Part model, mm, in its own coordinate system. Coordinates: 2 decimals unless noted, no trailing zeros. Order: outer loops, then holes, each group sorted by start corner. A loop starts at its lowest first (then second) coordinate and runs counter-clockwise, first axis right, second up.
```python
from build123d import *

# Parameters (mm, degrees)
SKETCH1_W           = 127
SKETCH1_H           = 63.5
BOSS_EXTRUDE1_DEPTH = 2.286
SKETCH2_R           = 3.3734375
CUT_EXTRUDE1_DEPTH  = 143.008717324
CHAMFER1_SIZE       = 20.32


with BuildPart() as part:
    # Sketch1 → Boss-Extrude1 (new body)
    with BuildSketch(Plane(origin=(0, 0, 0), x_dir=(1, 0, 0), z_dir=(0, 1, 0))):
        with Locations((63.5, 31.75)):
            Rectangle(SKETCH1_W, SKETCH1_H)
    extrude(amount=BOSS_EXTRUDE1_DEPTH)

    # Sketch2 → Cut-Extrude1 (cut, through all)
    with BuildSketch(Plane(origin=(0, 2.286, 0), x_dir=(1, 0, 0), z_dir=(0, 1, 0))):
        with Locations(Location((25.4, 25.4, 0), (0, 0, 270))):
            Circle(SKETCH2_R)
        with Locations(Location((101.6, 25.4, 0), (0, 0, 270))):
            Circle(SKETCH2_R)
    extrude(amount=-CUT_EXTRUDE1_DEPTH, mode=Mode.SUBTRACT)

    # Chamfer1
    chamfer1_edges = [part.edges().sort_by_distance(p)[0] for p in [
        (0, 1.143, -63.5),
        (127, 1.143, -63.5),
    ]]
    chamfer(chamfer1_edges, length=CHAMFER1_SIZE)


solid = part.part
```
(1) Slice it at A-A, the plane x = 101.6. Give the cut face in (y, z).
(2) Drop a flat-ended pin along its axis: pin 1 (9 mm diameter, centred on x = 25.4, z = -25.4, fed in from -Y). Give the stop position or say it passes through.
(3) Slice it at B-B, the plane z = -25.4. Give the cut face in (x, y), then the cut area to 3 significant figures.
(4) Slice it at D-D, the plane z = -47. Give the cut face in (x, y).
(5) Slice it at C-C, the plane y = 0.45. Give the cut face in (x, z), then the cut area to 3 significant figures.
(6) Pull direction Z, two halves, no side cores. Call faces 1 (the face through (63, 1, 0)), 2 (the face through (10.3, 1.13, -53.48)), 3 (the face through (63, 2.286, -32)), 4 (the face through (25.55, 1.16, -28.77)): +Z half, -Z half, draft (parallel to the pull), parting line (faces both ways), or undercut.
(7) Probe line 1 (X direction, y = 0.7, z = -25.4); line 2 (X direction, y = 1.6, z = -23); line 3 (Z direction, x = 100.5, y = 2). List the from-to ranges inside material, lowest first.
Here are the results:
1. outline: (0, -63.5) - (2.29, -63.5) - (2.29, -28.77) - (0, -28.77) - close; (0, -22.03) - (2.29, -22.03) - (2.29, 0) - (0, 0) - close
2. pin 1: stops at y = 0
3. outline: (0, 0) - (22.03, 0) - (22.03, 2.29) - (0, 2.29) - close; (28.77, 0) - (98.23, 0) - (98.23, 2.29) - (28.77, 2.29) - close; (104.97, 0) - (127, 0) - (127, 2.29) - (104.97, 2.29) - close
3. area: 259 mm2
4. outline: (3.82, 0) - (123.18, 0) - (123.18, 2.29) - (3.82, 2.29) - close
5. outline: (0, -43.18) - (20.32, -63.5) - (106.68, -63.5) - (127, -43.18) - (127, 0) - (0, 0) - close; hole circle Ø6.75 at (25.4, -25.4); hole circle Ø6.75 at (101.6, -25.4)
5. area: 7,580 mm2
6. face 1: +Z half
6. face 2: -Z half
6. face 3: draft
6. face 4: undercut
7. line 1: x = 0 to 22.03, 28.77 to 98.23, 104.97 to 127
7. line 2: x = 0 to 23.03, 27.77 to 99.23, 103.97 to 127
7. line 3: z = -63.5 to -28.59, -22.21 to 0
